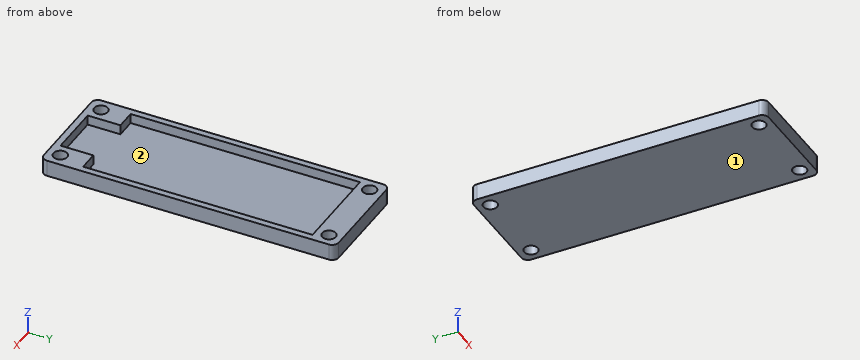
from build123d import *

# Parameters (mm, degrees)
EXTRUDE001_DEPTH = 3
SKETCH_W         = 32
SKETCH_H         = 90
SKETCH_R         = 2.1
EXTRUDE_DEPTH    = 5
FILLET_R         = 2


with BuildPart() as extrude001:
    # Sketch001 (on Face5 of Fillet) → Extrude001 (new body)
    with BuildSketch(Plane.XY.offset(5)):
        Polygon((14, 37), (14, -33), (8, -33), (8, -43), (-8, -43), (-8, -33), (-14, -33), (-14, 37), align=None)
    extrude(amount=-EXTRUDE001_DEPTH)


with BuildPart() as cut:
    # Sketch → Extrude (new body)
    with BuildSketch(Plane.XY):
        Rectangle(SKETCH_W, SKETCH_H)
        with Locations((-12, 41)):
            Circle(SKETCH_R, mode=Mode.SUBTRACT)
        with Locations((12, 41)):
            Circle(SKETCH_R, mode=Mode.SUBTRACT)
        with Locations((-12, -41)):
            Circle(SKETCH_R, mode=Mode.SUBTRACT)
        with Locations((12, -41)):
            Circle(SKETCH_R, mode=Mode.SUBTRACT)
    extrude(amount=EXTRUDE_DEPTH)

    # Fillet
    fillet_edges = [cut.edges().sort_by_distance(p)[0] for p in [
        (-16, 45, 2.5),
        (16, 45, 2.5),
        (16, -45, 2.5),
        (-16, -45, 2.5),
    ]]
    fillet(fillet_edges, radius=FILLET_R)

    # Cut: cut Extrude001
    add(extrude001.part, mode=Mode.SUBTRACT)


solid = cut.part
Input: part model. Units: mm. Frame: model coordinates. Face numbers are marked on the shaded views. Give positions to 0.01 mm unless a question says otherwise; leave off trailing zeros. Write each loop counter-clockwise with the first axis right and the second up, starting at its lowest first coordinate (ties: lowest second). Pieces come first, ordered by that corner, then holes. Notation, with made-up numbers: M 72.5,0 L 93.5,0 A25 cw 93.5,18 Z; hole C 65,13.25 d8. An arc over 180 degrees is marked long. Write item = value, one per line. Start each with the question number.
1) First-contact query: pin 1 Ø6 at (x, y) = (-4.5, 16) entering from +Z. Flat tip, straight axial feed; report the tip coordinate or a pass-through.
2) Material intervals for line 1 along Y through (x, z) = (12, 1.8); line 2 along Y through (x, z) = (12, 3.55); line 3 along X through (y, z) = (13, 2.95), sorted ascending. Write a range as [from, to].
3) Cut plane D-D on x = 1. Return the cut outline in (y, z), then the cut area to 3 significant figures.
4) Cut plane C-C on y = 41. Return the cut outline in (x, z).
5) Draft query along X for the marked faces 1 and 2. Return one class per face: +X half, -X half, draft (parallel to the pull), parting line (faces both ways), or undercut.
6) Cut plane A-A on y = -41. Return the cut outline in (x, z).
7) Cut plane B-B on x = 12. Return the cut outline in (y, z), then the cut area to 3 significant figures.
Solved:
q1.pin_1 = 2
q2.line_1 = [-45, -43.1], [-38.9, 38.9], [43.1, 45]
q2.line_2 = [-45, -43.1], [-38.9, -33], [37, 38.9], [43.1, 45]
q2.line_3 = [-16, -14], [14, 16]
q3.outline = M -45,0 L 45,0 L 45,5 L 37,5 L 37,2 L -43,2 L -43,5 L -45,5 Z
q3.area = 210 mm2
q4.outline = M -16,0 L -14.1,0 L -14.1,5 L -16,5 Z; M -9.9,0 L 9.9,0 L 9.9,5 L -9.9,5 Z; M 14.1,0 L 16,0 L 16,5 L 14.1,5 Z
q5.face_1 = draft
q5.face_2 = undercut
q6.outline = M -16,0 L -14.1,0 L -14.1,5 L -16,5 Z; M -9.9,0 L 9.9,0 L 9.9,5 L 8,5 L 8,2 L -8,2 L -8,5 L -9.9,5 Z; M 14.1,0 L 16,0 L 16,5 L 14.1,5 Z
q7.outline = M -45,0 L -43.1,0 L -43.1,5 L -45,5 Z; M -38.9,0 L 38.9,0 L 38.9,5 L 37,5 L 37,2 L -33,2 L -33,5 L -38.9,5 Z; M 43.1,0 L 45,0 L 45,5 L 43.1,5 Z
q7.area = 198 mm2
